from build123d import *

# Parameters (mm, degrees)
SKETCH021_W     = 30.610564
SKETCH021_H     = 3
POCKET_DEPTH    = 3.001
SKETCH023_R     = 2
POCKET001_DEPTH = 3.001


with BuildPart() as part:
    # Sketch021 → Revolution008 (revolve)
    with BuildSketch(Plane.YZ):
        with Locations((-15.305282, 63.385058)):
            Rectangle(SKETCH021_W, SKETCH021_H)
    revolve(axis=Axis((0, 0, 0), (0, 0, 1)))

    # Sketch022 (on Face1 of Revolution008) → Pocket (cut, through all)
    with BuildSketch(Plane(origin=(0, 0, 64.885058), x_dir=(0, -1, 0), z_dir=(0, 0, 1))):
        with BuildLine():
            Line((-2.378645, 11.760677), (5.571355, 11.760677))
            Line((5.571355, 11.760677), (5.571355, -12.639323))
            Line((5.571355, -12.639323), (-2.378645, -12.639323))
            ThreePointArc((-7.328645, -7.689323), (-5.878824, -11.189501), (-2.378645, -12.639323))
            Line((-7.328645, -7.689323), (-7.328645, 6.810677))
            ThreePointArc((-2.378645, 11.760677), (-5.878824, 10.310856), (-7.328645, 6.810677))
        make_face()
    extrude(amount=-POCKET_DEPTH, mode=Mode.SUBTRACT)

    # Sketch023 (on Face1 of Pocket) → Pocket001 (cut, through all)
    with BuildSketch(Plane(origin=(0, 0, 64.885058), x_dir=(0, -1, 0), z_dir=(0, 0, 1))):
        with Locations((-17.273551, -9.97289)):
            Circle(SKETCH023_R)
        with Locations((17.273551, -9.97289)):
            Circle(SKETCH023_R)
        with Locations((0, 19.945779)):
            Circle(SKETCH023_R)
    extrude(amount=-POCKET001_DEPTH, mode=Mode.SUBTRACT)


solid = part.part
Here's how the part is built. I have some questions about the finished solid (model axes, mm). A direction names the side the tool comes from. Give positions to 0.01 mm unless a question says otherwise; leave off trailing zeros. Order: outer loops, then holes, each group sorted by start corner. A loop starts at its lowest first (then second) coordinate and runs counter-clockwise, first axis right, second up. Notation, with made-up numbers: M -28.5,56.25 L 15.5,56.25 A16 cw 15.5,71.25 Z; hole C -20,-17.5 d9. An arc over 180 degrees is marked long. Answer as a JSON object with one key per item and string values. Group by question number.
1) Suppose I cut it at A-A, the plane x = 0. Write out the boundary of the cut face in (y, z).
2) Suppose I cut it at C-C, the plane x = -9. Write out the boundary of the cut face in (y, z), plus the area to 3 significant figures.
3) I'm going to push flat-ended pins straight in: pin 1 Ø0.9 at (y, z) = (-0.5, 63) entering from -X; pin 2 Ø3.5 at (x, y) = (19.95, 0) entering from -Z; pin 3 Ø1.5 at (x, z) = (-5.5, 63) entering from +Y. Where does each tip first touch, or does it pass through?
4) We'd pull the mould along Y, two halves only. Please class faces 3 (the cylindrical face through (-8.62, -15.8, 63.41)), 4 (the cylindrical face through (1.35, 30.58, 63.41)), 5 (the flat face through (0, -6, 64.885)): pulls with the +Y half, pulls with the -Y half, needs draft (parallel to the pull), parting line crosses it, or undercut.
5) Suppose I cut it at B-B, the plane y = 0. Write out the boundary of the cut face in (x, z).
6) On a 3-axis mill with a long thin cutter (end or side, diameter ignored), from which of +Z, -Z, +X, -X, +Y, -Y can I reach the whole of each face in a straight line? I mean faces 1 (the flat face through (11.761, -2, 63)), 2 (the flat face through (0, -6, 61.885)). Say none if no direction works.
7) Please list where these lines run through material, in increasing order: L1, parallel to X at y = 0, z = 63.75; L2, parallel to Y at x = 6.5, z = 62.9; L3, parallel to Y at x = -6, z = 64.1. Write a range as [from, to].
8) Suppose I cut it at D-D, the plane z = 62.5. Write out the boundary of the cut face in (x, y), plus the area to 3 significant figures.
Results found:
{
 "1": {"outline": "M -30.61,61.89 L -5.57,61.89 L -5.57,64.89 L -30.61,64.89 Z; M 7.33,61.89 L 30.61,61.89 L 30.61,64.89 L 7.33,64.89 Z"},
 "2": {"outline": "M -29.26,61.89 L -19.02,61.89 L -19.02,64.89 L -29.26,64.89 Z; M -15.53,61.89 L -5.57,61.89 L -5.57,64.89 L -15.53,64.89 Z; M 7.15,61.89 L 15.53,61.89 L 15.53,64.89 L 7.15,64.89 Z; M 19.02,61.89 L 29.26,61.89 L 29.26,64.89 L 19.02,64.89 Z", "area": "116 mm²"},
 "3": {"pin 1": "x = -30.61", "pin 2": "through", "pin 3": "y = 30.24"},
 "4": {"face 3": "undercut", "face 4": "parting line crosses it", "face 5": "needs draft"},
 "5": {"outline": "M -30.61,61.89 L -12.64,61.89 L -12.64,64.89 L -30.61,64.89 Z; M 11.76,61.89 L 17.95,61.89 L 17.95,64.89 L 11.76,64.89 Z; M 21.95,61.89 L 30.61,61.89 L 30.61,64.89 L 21.95,64.89 Z"},
 "6": {"face 1": "+Z, -Z", "face 2": "-Z, +X, -X, +Y, -Y"},
 "7": {"L1": "[-30.61, -12.64], [11.76, 17.95], [21.95, 30.61]", "L2": "[-29.91, -5.57], [7.33, 29.91]", "L3": "[-30.02, -5.57], [7.33, 30.02]"},
 "8": {"outline": "C 0,0 d61.22; hole M -12.64,-5.57 L 11.76,-5.57 L 11.76,2.38 A4.95 ccw 6.81,7.33 L -7.69,7.33 A4.95 ccw -12.64,2.38 Z; hole C -9.97,-17.27 d4; hole C -9.97,17.27 d4; hole C 19.95,0 d4", "area": "2,600 mm²"}
}
